Verification items for the finished model (mm, model axes). A direction names the side the tool comes from. Round coordinates to 2 decimals unless told otherwise and drop trailing zeros. Loops run counter-clockwise (first coordinate to the right, second up) from the corner with the lowest first, then second, coordinate; pieces in that order, holes last. Notation, with made-up numbers: (47.5, 74.25) -> (98.5, 74.25) arc R18 ccw to (98.5, 88.25) -> close; hole circle Ø3 at (-5.75, 85.5). An arc over 180 degrees is marked (long way). Write item = value, one per line. Start each with the question number.
```python
from build123d import *

# Parameters (mm, degrees)
F1_DEPTH = 60
F2_W     = 91
F2_H     = 40
F3_DEPTH = 20
F4_R     = 4.3757639441
F5_DEPTH = 2.5
F7_DEPTH = 120.001
F8_R     = 10


with BuildPart() as f1:
    # F0 (on Right) → F1 (new body, symmetric)
    with BuildSketch(Plane.YZ):
        Polygon((35, 0), (0, 60.6217782649), (-35, 0), align=None)
    extrude(amount=F1_DEPTH, both=True)

    # F2 (on face) → F3 (cut)
    with BuildSketch(Plane(origin=(0, -26.25, 15.1554445662), x_dir=(1, 0, 0), z_dir=(0, -0.8660254038, 0.5))):
        with Locations((0, 32.5)):
            Rectangle(F2_W, F2_H)
    extrude(amount=-F3_DEPTH, mode=Mode.SUBTRACT)

    # F4 (on face) → F5 (join)
    with BuildSketch(Plane(origin=(0, -26.25, 15.1554445662), x_dir=(1, 0, 0), z_dir=(0, -0.8660254038, 0.5))):
        Polygon((-16.9133506715, 6.9602951407), (-32.6403528452, 6.9602951407), (-18.8582409173, -12.9176480696), (-3.2289559022, -12.9176480696), align=None)
        Polygon((2.3815555032, 6.9602951407), (-13.3497389033, 6.9602951407), (0.334655866, -12.9176480696), (16.0643365234, -12.9176480696), align=None)
        with BuildLine():
            Line((15.8933419219, 6.9602951407), (6.0318070464, 6.9602951407))
            Line((6.0318070464, 6.9602951407), (11.8799349226, -1.2600759071))
            ThreePointArc((11.8799349226, -1.2600759071), (12.0659931402, 3.7389977797), (15.8933419219, 6.9602951407))
        make_face()
        with Locations((17.6157766381, 1.0294436968)):
            Circle(F4_R)
        with BuildLine():
            Line((23.2472105613, -1.5060507656), (29.0346425027, 6.9602951407))
            Line((29.0346425027, 6.9602951407), (19.3382113542, 6.9602951407))
            ThreePointArc((19.3382113542, 6.9602951407), (23.2228792092, 3.6183007725), (23.2472105613, -1.5060507656))
        make_face()
        with BuildLine():
            Line((13.5719669058, -3.6384662263), (17.7627429366, -9.5291947946))
            Line((17.7627429366, -9.5291947946), (22.0228294821, -3.29717917))
            ThreePointArc((22.0228294821, -3.29717917), (17.8649865963, -5.1414293855), (13.5719669058, -3.6384662263))
        make_face()
    extrude(amount=F5_DEPTH)

    # F6 (on face) → F7 (cut, through all)
    with BuildSketch(Plane(origin=(-60, 0, 0), x_dir=(0, -1, 0), z_dir=(-1, 0, 0))):
        Polygon((10, 0), (0, 17.3205080757), (-10, 0), align=None)
    extrude(amount=-F7_DEPTH, mode=Mode.SUBTRACT)

    # F8
    f8_edges = [f1.edges().sort_by_distance(p)[0] for p in [
        (52.75, 0, 60.621778),
        (-52.75, 0, 60.621778),
        (-60, -17.5, 30.310889),
        (60, 17.5, 30.310889),
        (60, -17.5, 30.310889),
        (-60, 17.5, 30.310889),
        (-60, -5, 8.660254),
        (-60, 5, 8.660254),
        (60, -5, 8.660254),
        (60, 5, 8.660254),
    ]]
    fillet(f8_edges, radius=F8_R)


solid = f1.part
```
(1) Access from +Z, -Z, +X, -X, +Y, -Y to the whole of each face (thin tool, end or side, straight path). Record for faces 5 (the flat face through (-0.7, 4.93, 8.78)), 6 (the flat face through (19.86, -30.55, 10.18)), 7 (the flat face through (-9.975, -28.876, 13.072)), 8 (the flat face through (1, 22, 0)), 9 (the cylindrical face through (58.254, 8.128, 11.952)).
(2) Scan lines: line 1 (Y direction, x = 42, z = 12.5); line 2 (X direction, y = 5, z = 35.5); line 3 (Y direction, x = 13.5, z = 9). Record each from-to range of solid material in increasing order. Write a range as [from, to].
(3) Section check A-A on x = -11.5. Enter the section's corners in (y, z), then the cut area to 3 significant figures.
(4) Section check B-B on x = 9. Enter the section's corners in (y, z), then the cut area to 3 significant figures.
(5) Depth check by flat-ended pin: pin 1 Ø6 at (x, z) = (21.5, 45) entering from -Y; pin 2 Ø2 at (x, z) = (11, 37) entering from -Y; pin 3 Ø12 at (y, z) = (-24.5, 25.5) entering from +X; pin 4 Ø6 at (x, z) = (41.5, 39) entering from +Y. Enter the tip coordinate at first touch or a pass-through.
(6) Draft check along Y on faces 1 (the cylindrical face through (-58.254, 8.429, 11.43)), 2 (the cylindrical face through (47.78, 0.15, 50.62)), 3 (the cylindrical face through (12.035, -25.48, 18.953)), 4 (the flat face through (1, -23, 0)). Enter one of: +Y half, -Y half, draft (parallel to the pull), parting line (faces both ways), or undercut.
Computed values:
q1.face_5 = -Z, +X, -X
q1.face_6 = +X, -Y
q1.face_7 = +Z
q1.face_8 = -Z, +X, -X, +Y, -Y
q1.face_9 = -Z, +X
q2.line_1 = [-27.78, -2.78], [2.78, 27.78]
q2.line_2 = [-59.84, -45.5], [45.5, 59.84]
q2.line_3 = [-29.8, -4.8], [4.8, 29.8]
q3.outline = (-35, 0) -> (-10, 0) -> (0, 17.32) -> (10, 0) -> (35, 0) -> (11.55, 40.62) -> (-2.68, 15.98) -> (-20, 25.98) -> (-22.77, 21.18) -> (-24.93, 22.43) -> (-26.28, 20.11) -> (-24.11, 18.86) -> (-26.7, 14.37) -> (-28.87, 15.62) -> (-34.87, 5.22) -> (-32.71, 3.97) -> close
q3.area = 1,300 mm²
q4.outline = (-35, 0) -> (-10, 0) -> (0, 17.32) -> (10, 0) -> (35, 0) -> (11.55, 40.62) -> (-2.68, 15.98) -> (-20, 25.98) -> (-22.77, 21.18) -> (-24.93, 22.43) -> (-27.02, 18.82) -> (-24.86, 17.57) -> (-27.58, 12.86) -> (-29.74, 14.11) -> (-34.87, 5.22) -> (-32.71, 3.97) -> close
q4.area = 1,300 mm²
q5.pin_1 = through
q5.pin_2 = 8.88
q5.pin_3 = 56.43
q5.pin_4 = 14.22
q6.face_1 = undercut
q6.face_2 = parting line
q6.face_3 = undercut
q6.face_4 = draft
